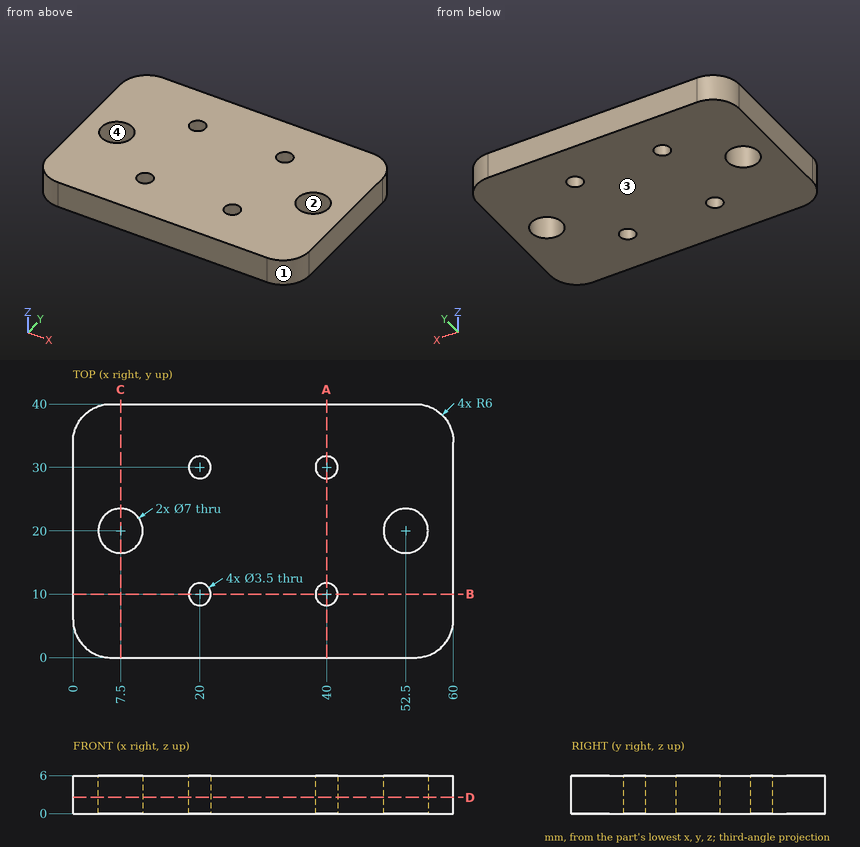
Check sheet for the drawn part. Datum: minimum x, y, z corner. Units: mm. Coordinates: 2 decimals unless noted, no trailing zeros. Write each loop counter-clockwise with the first axis right and the second up, starting at its lowest first coordinate (ties: lowest second). Pieces come first, ordered by that corner, then holes. Notation, with made-up numbers: (-26.75, 81.5) - (21.25, 81.5) arc R25 cw to (21.25, 96.5) - close; hole circle Ø4 at (-22, 76.25). An arc over 180 degrees is marked (long way). Answer as a JSON object with one key per item and string values.
(1) Cross-section at B-B on y = 10. Record the cut outline in (x, z).
Report:
{"outline": "(0, 0) - (18.25, 0) - (18.25, 6) - (0, 6) - close; (21.75, 0) - (38.25, 0) - (38.25, 6) - (21.75, 6) - close; (41.75, 0) - (60, 0) - (60, 6) - (41.75, 6) - close"}
(2) Cross-section at A-A on x = 40. Record the cut outline in (y, z), plus the area to 3 significant figures.
Report:
{"outline": "(0, 0) - (8.25, 0) - (8.25, 6) - (0, 6) - close; (11.75, 0) - (28.25, 0) - (28.25, 6) - (11.75, 6) - close; (31.75, 0) - (40, 0) - (40, 6) - (31.75, 6) - close", "area": "198 mm^2"}
(3) Thickness scan on line 1 along Y through (x, z) = (20, 4.3); line 2 along X through (y, z) = (9, 1.45); line 3 along X through (y, z) = (31.5, 3.7). Record the ranges inside material, lowest first.
Report:
{"line 1": "0 to 8.25, 11.75 to 28.25, 31.75 to 40", "line 2": "0 to 18.56, 21.44 to 38.56, 41.44 to 60", "line 3": "0 to 19.1, 20.9 to 39.1, 40.9 to 60"}
(4) Cross-section at D-D on z = 2.55. Record the cut outline in (x, y).
Report:
{"outline": "(0, 6) arc R6 ccw to (6, 0) - (54, 0) arc R6 ccw to (60, 6) - (60, 34) arc R6 ccw to (54, 40) - (6, 40) arc R6 ccw to (0, 34) - close; hole circle Ø7 at (7.5, 20); hole circle Ø3.5 at (20, 10); hole circle Ø3.5 at (20, 30); hole circle Ø3.5 at (40, 10); hole circle Ø3.5 at (40, 30); hole circle Ø7 at (52.5, 20)"}
(5) Mould release check, pull along X, two halves, no side actions. Record for the marked faces 1, 2, 3 and 4: pulls with the +X half, pulls with the -X half, needs draft (parallel to the pull), parting line crosses it, or undercut.
Report:
{"face 1": "pulls with the +X half", "face 2": "undercut", "face 3": "needs draft", "face 4": "undercut"}
(6) Gauge pin test, flat end, axial feed: pin 1 Ø4 at (x, y) = (7.5, 20) entering from +Z. Record the tip position at first contact, or that the pin passes through.
Report:
{"pin 1": "through"}
(7) Cross-section at C-C on x = 7.5. Record the cut outline in (y, z), plus the area to 3 significant figures.
Report:
{"outline": "(0, 0) - (16.5, 0) - (16.5, 6) - (0, 6) - close; (23.5, 0) - (40, 0) - (40, 6) - (23.5, 6) - close", "area": "198 mm^2"}
